Input: part model. Units: mm. Frame: model coordinates. Coordinates: 2 decimals unless noted, no trailing zeros. Order: outer loops, then holes, each group sorted by start corner. A loop starts at its lowest first (then second) coordinate and runs counter-clockwise, first axis right, second up. Notation, with made-up numbers: M 61,-7 L 92,-7 A30 cw 92,18 Z; hole C 49.5,64.5 d6. An arc over 180 degrees is marked long. Answer in a Markdown table with one row per item.
Autodesk Inventor part; units mm, degrees
ref_plane "YZ Plane" through (0, 0, 0) normal (1, 0, 0) x (0, 1, 0)
ref_plane "XZ Plane" through (0, 0, 0) normal (0, 1, 0) x (-1, 0, 0)
ref_plane "XY Plane" through (0, 0, 0) normal (0, 0, 1) x (1, 0, 0)
sketch "Sketch1" plane through (0, 0, 0) normal (0, 1, 0) x (-1, 0, 0)
  circle A0 centre (0, 0) radius 1.5
  dimension "d0" = 3
extrude "Extrusion1" add sketch "Sketch1" along normal blind 30
chamfer "Chamfer1" distance 0.25 angle 45 2 edges at (1.5, 30, 0) (1.5, 0, 0)
sketch "Sketch2" plane through (0, 0, 0) normal (0, -1, 0) x (1, 0, 0)
  circle A0 centre (0, 0) radius 0.75
  dimension "d6" = 1.5
extrude "Extrusion2" cut sketch "Sketch2" against normal blind 30
properties part number "pin_3_30"
1) Material intervals for probe 1 along Z at (x, y) = (0, 10.75); probe 2 along X at (y, z) = (19.5, 0.35); probe 3 along X at (y, z) = (18.5, -0.5), sorted ascending.
Resolved:
| item | result |
|---|---|
| probe 1 | z = -1.5 to -0.75, 0.75 to 1.5 |
| probe 2 | x = -1.46 to -0.66, 0.66 to 1.46 |
| probe 3 | x = -1.41 to -0.56, 0.56 to 1.41 |
2) Cut plane C-C, the plane y = 12.25. Output: boundary loops of the cut face in (x, z), and give its area (3 significant figures).
Resolved:
| item | result |
|---|---|
| outline | C 0,0 d3; hole C 0,0 d1.5 |
| area | 5.30 mm2 |
3) Mould query, pull axis Z, two halves, no side actions, for faces 1 (the face through (-0.75, 14.79, 0.03)), 2 (the face through (1.5, 14.79, -0.07)), 3 (the face through (-1, 30, 0)). Classes: +Z half, -Z half, draft (parallel to the pull), parting line (faces both ways), or undercut.
Resolved:
| item | result |
|---|---|
| face 1 | undercut |
| face 2 | parting line |
| face 3 | draft |
4) Contact query for flat-ended pins moving along their axis: pin 1 (1 mm diameter, centred on x = 1, z = -1, fed in from -Y); pin 2 (1 mm diameter, centred on x = 1, y = 6, fed in from -Z). Output: stop coordinate, or through.
Resolved:
| item | result |
|---|---|
| pin 1 | stops at y = 0 |
| pin 2 | stops at z = -1.41 |
5) Cut plane B-B, the plane z = 0. Output: boundary loops of the cut face in (x, y).
Resolved:
| item | result |
|---|---|
| outline | M -1.5,0.25 L -1.25,0 L -0.75,0 L -0.75,30 L -1.25,30 L -1.5,29.75 Z; M 0.75,0 L 1.25,0 L 1.5,0.25 L 1.5,29.75 L 1.25,30 L 0.75,30 Z |
6) Cut plane A-A, the plane x = 0. Output: boundary loops of the cut face in (y, z), and give its area (3 significant figures).
Resolved:
| item | result |
|---|---|
| outline | M 0,-1.25 L 0.25,-1.5 L 29.75,-1.5 L 30,-1.25 L 30,-0.75 L 0,-0.75 Z; M 0,0.75 L 30,0.75 L 30,1.25 L 29.75,1.5 L 0.25,1.5 L 0,1.25 Z |
| area | 44.9 mm2 |
